Geometry: see drawing. Coordinates: mm, zero at the bounding-box minimum. A direction names the side the tool comes from. Coordinates: 2 decimals unless noted, no trailing zeros. Write each loop counter-clockwise with the first axis right and the second up, starting at its lowest first coordinate (ties: lowest second). Pieces come first, ordered by that corner, then holes. Notation, with made-up numbers: M 24,-8 L 46,-8 A31 cw 46,29 Z; hole C 61,34 d5. An arc over 180 degrees is marked long. Write item = value, one per line. Start each with the question number.
1. Section query C-C (y = 29). Output: boundary loops of the cut face in (x, z).
2. Section query B-B (x = 63). Output: boundary loops of the cut face in (y, z), then the cut area to 3 significant figures.
3. Access query for the marked faces 1 and 2. Directions: +Z, -Z, +X, -X, +Y, -Y. A direction counts if a zero-diameter tool reaches every point of the face in a straight line with its end or side. Return the directions, or none.
4. Pull-direction query (X, two-part tool) for the marked faces 3, 4 and 5; classes: pulls with the +X half, pulls with the -X half, needs draft (parallel to the pull), parting line crosses it, or undercut.
5. Section query A-A (z = 6). Output: boundary loops of the cut face in (x, y), then the cut area to 3 significant figures.
6. Pin query (flat end, axial travel): pin 1 Ø3 at (x, z) = (47, 5) entering from -Y. Return the tip coordinate at first contact, or that it passes through.
7. Line query: line 1 along X through (y, z) = (10.5, 3); line 2 along Z through (x, y) = (9.5, 64.5). Output: solid intervals per line, ascending.
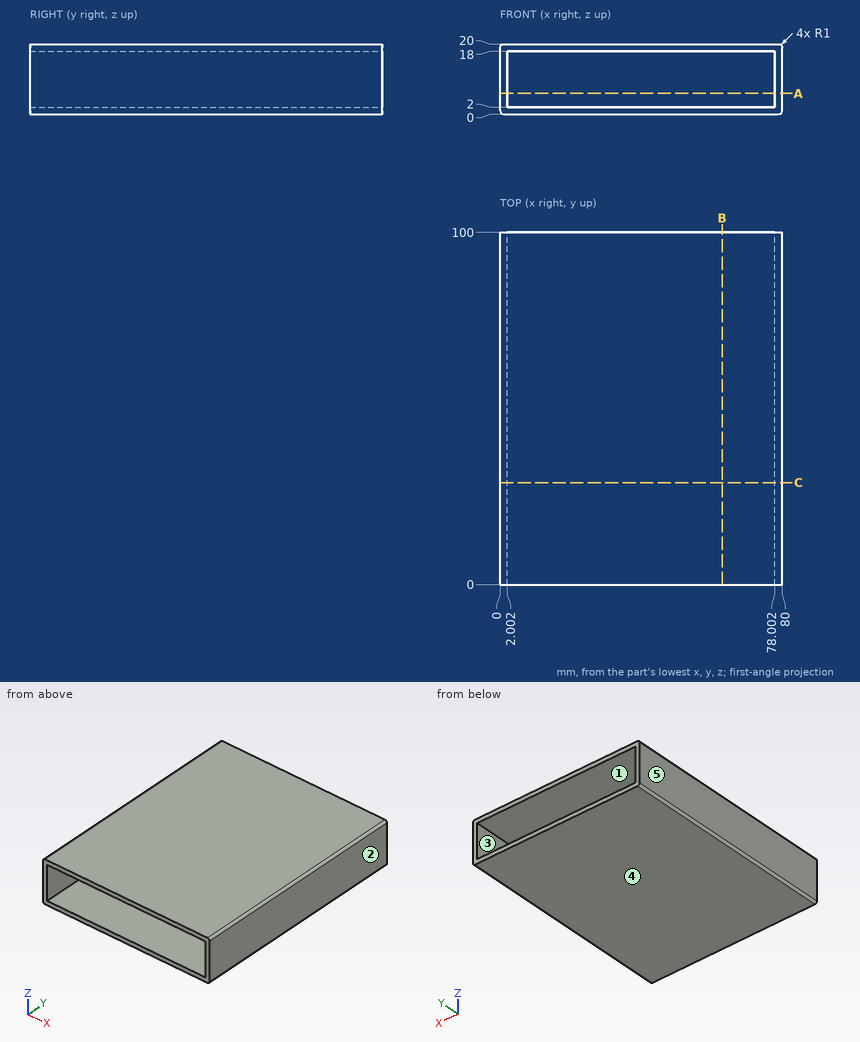
Results are:
q1.outline = M 0,1 A1 ccw 1,0 L 79,0 A1 ccw 80,1 L 80,19 A1 ccw 79,20 L 1,20 A1 ccw 0,19 Z; hole M 2,2 L 78,2 L 78,18 L 2,18 Z
q2.outline = M 0,0 L 100,0 L 100,2 L 0,2 Z; M 0,18 L 100,18 L 100,20 L 0,20 Z
q2.area = 400 mm^2
q3.face_1 = +Y, -Y
q3.face_2 = +Z, -Z, +X, +Y, -Y
q4.face_3 = undercut
q4.face_4 = needs draft
q4.face_5 = pulls with the -X half
q5.outline = M 0,0 L 2,0 L 2,100 L 0,100 Z; M 78,0 L 80,0 L 80,100 L 78,100 Z
q5.area = 400 mm^2
q6.pin_1 = through
q7.line_1 = 0 to 2, 78 to 80
q7.line_2 = 0 to 2, 18 to 20
